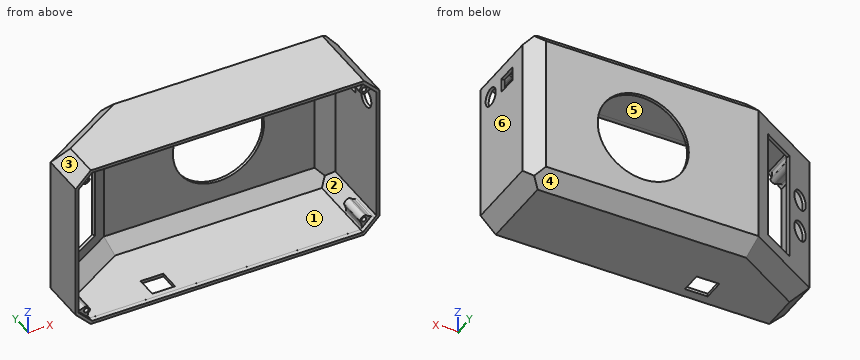
```python
from build123d import *

# Parameters (mm, degrees)
BOSS_EXTRUDE1_DEPTH = 110
CHAMFER1_SIZE       = 10
CHAMFER2_SIZE       = 10
SHELL2_T            = -2
SKETCH2_W           = 25
SKETCH2_H           = 72
CUT_EXTRUDE2_DEPTH  = 90
SKETCH4_R           = 6.5
CUT_EXTRUDE3_DEPTH  = 90
SKETCH5_R           = 1.5
BOSS_EXTRUDE2_DEPTH = 22
FILLET2_R           = 1
CUT_EXTRUDE4_DEPTH  = 3
SKETCH7_R           = 30
CUT_EXTRUDE5_DEPTH  = 61
SKETCH9_R           = 6
SKETCH9_W           = 9.2
SKETCH9_H           = 13
CUT_EXTRUDE6_DEPTH  = 48
SKETCH10_W          = 15
SKETCH10_H          = 14
CUT_EXTRUDE7_DEPTH  = 48


with BuildPart() as part:
    # Sketch1 → Boss-Extrude1 (new body)
    with BuildSketch(Plane.XY):
        Polygon((-200, 30), (-150, 60), (0, 60), (0, 0), (-200, 0), align=None)
    extrude(amount=BOSS_EXTRUDE1_DEPTH)

    # Chamfer1
    chamfer1_edges = [part.edges().sort_by_distance(p)[0] for p in [
        (-175, 45, 110),
        (-200, 15, 110),
        (0, 30, 110),
        (-200, 15, 0),
        (-175, 45, 0),
        (-75, 60, 0),
        (0, 30, 0),
        (-75, 60, 110),
    ]]
    chamfer(chamfer1_edges, length=CHAMFER1_SIZE)

    # Chamfer2
    chamfer2_edges = [part.edges().sort_by_distance(p)[0] for p in [
        (0, 60, 55),
    ]]
    chamfer(chamfer2_edges, length=CHAMFER2_SIZE)

    # Shell2
    shell2_openings = [part.faces().sort_by_distance(p)[0] for p in [
        (-100, 0, 55),
    ]]
    offset(amount=SHELL2_T, openings=shell2_openings, kind=Kind.INTERSECTION)

    # Sketch2 → Cut-Extrude2 (cut)
    with BuildSketch(Plane(origin=(-66.176470588, 110.294117647, 0), x_dir=(0.8574929257125443, 0.5144957554275263, 0), z_dir=(-0.5144957554275263, 0.8574929257125443, 0))):
        with Locations((-120.89691226, -53.994862886)):
            Rectangle(SKETCH2_W, SKETCH2_H)
    extrude(amount=-CUT_EXTRUDE2_DEPTH, mode=Mode.SUBTRACT)

    # Sketch4 → Cut-Extrude3 (cut)
    with BuildSketch(Plane(origin=(-66.176470588, 110.294117647, 0), x_dir=(0.8574929257125443, 0.5144957554275263, 0), z_dir=(-0.5144957554275263, 0.8574929257125443, 0))):
        with Locations(Location((-145.210771321, -43.863127818, 0), (0, 0, 180))):
            Circle(SKETCH4_R)
        with Locations(Location((-145.284101168, -65.939492282, 0), (0, 0, 180))):
            Circle(SKETCH4_R)
    extrude(amount=-CUT_EXTRUDE3_DEPTH, mode=Mode.SUBTRACT)

    # Sketch5 → Boss-Extrude2 (add)
    # profile 1 of 4: a face of its own
    with BuildSketch(Plane.XZ):
        with BuildLine():
            Line((-9.247397896, 106.757043705), (-3.256064459, 100.483765165))
            ThreePointArc((-3.256064459, 100.483765165), (-5.744873038, 99.736713828), (-7.870281401, 98.241757931))
            ThreePointArc((-7.870281401, 98.241757931), (-10.292221795, 99.429108259), (-11.636574356, 101.767550533))
            ThreePointArc((-11.636574356, 101.767550533), (-10.323587398, 104.205602893), (-9.247397896, 106.757043705))
        make_face()
        with Locations((-8.511299496, 101.440505433)):
            Circle(SKETCH5_R, mode=Mode.SUBTRACT)
    # profile 2 of 4: a face of its own
    with BuildSketch(Plane.XZ):
        with BuildLine():
            Line((-10.039510209, 2.683192712), (-3.513368166, 9.046181203))
            ThreePointArc((-3.513368166, 9.046181203), (-5.632030744, 9.88127065), (-7.41571196, 11.29710497))
            ThreePointArc((-7.41571196, 11.29710497), (-9.918845287, 10.389628717), (-11.372165694, 8.158698553))
            ThreePointArc((-11.372165694, 8.158698553), (-10.188591886, 5.546835518), (-10.039510209, 2.683192712))
        make_face()
        with Locations((-8.560298278, 8.510476998)):
            Circle(SKETCH5_R, mode=Mode.SUBTRACT)
    # profile 3 of 4: a face of its own
    with BuildSketch(Plane.XZ):
        with BuildLine():
            Line((-190.1639185, 107.037062189), (-196.90252996, 100.401487601))
            ThreePointArc((-196.90252996, 100.401487601), (-194.442462904, 99.997388644), (-192.214833899, 98.878060765))
            ThreePointArc((-192.214833899, 98.878060765), (-190.200311855, 99.737450982), (-188.807968894, 101.428081542))
            ThreePointArc((-188.807968894, 101.428081542), (-190.20827937, 104.057949981), (-190.1639185, 107.037062189))
        make_face()
        with Locations((-191.50742986, 101.422355381)):
            Circle(SKETCH5_R, mode=Mode.SUBTRACT)
    # profile 4 of 4: a face of its own
    with BuildSketch(Plane.XZ):
        with BuildLine():
            Line((-190.456179178, 3.22389745), (-196.869032371, 9.61475183))
            ThreePointArc((-196.869032371, 9.61475183), (-194.424366222, 10.415493615), (-192.013666474, 11.313328071))
            ThreePointArc((-192.013666474, 11.313328071), (-189.789786951, 9.928723292), (-188.777999187, 7.512309411))
            ThreePointArc((-188.777999187, 7.512309411), (-190.165240448, 5.582610921), (-190.456179178, 3.22389745))
        make_face()
        with Locations((-191.356454927, 8.42171973)):
            Circle(SKETCH5_R, mode=Mode.SUBTRACT)
    extrude(amount=-BOSS_EXTRUDE2_DEPTH)

    # Fillet2
    fillet2_edges = [part.edges().sort_by_distance(p)[0] for p in [
        (-196.80570876, 11, 9.634135884),
        (-190.464527553, 11, 3.292954677),
        (-188.777999187, 11, 7.512309411),
        (-192.013666474, 11, 11.313328071),
        (-10.024061604, 11, 2.80436552),
        (-3.72900082, 11, 9.099426304),
        (-7.41571196, 11, 11.29710497),
        (-11.372165694, 11, 8.158698553),
        (-196.772588823, 11, 100.398984052),
        (-190.174781799, 11, 106.996791076),
        (-192.214833899, 11, 98.878060765),
        (-188.807968894, 11, 101.428081542),
        (-3.305525067, 11, 100.477097942),
        (-9.339081083, 11, 106.510653959),
        (-11.636574356, 11, 101.767550533),
        (-7.870281401, 11, 98.241757931),
    ]]
    fillet(fillet2_edges, radius=FILLET2_R)

    # Sketch6 → Cut-Extrude4 (cut)
    with BuildSketch(Plane.XZ):
        Polygon((-198.003014977, 10.842085531), (-189.211900871, 1.9947291), (-10.828081787, 1.9947291), (-2.004701189, 10.828504844), (-2.004701189, 99.205715336), (-10.87289136, 108.000350983), (-189.173255871, 108.000350983), (-198.003014977, 99.184415132), align=None)
    extrude(amount=-CUT_EXTRUDE4_DEPTH, mode=Mode.SUBTRACT)

    # Sketch7 → Cut-Extrude5 (cut)
    with BuildSketch(Plane(origin=(0, 60, 0), x_dir=(1, 0, 0), z_dir=(0, 1, 0))):
        with Locations(Location((-74.048474832, -53.651868822, 0), (0, 0, 180))):
            Circle(SKETCH7_R)
    extrude(amount=-CUT_EXTRUDE5_DEPTH, mode=Mode.SUBTRACT)

    # Sketch9 → Cut-Extrude6 (cut)
    with BuildSketch(Plane(origin=(0, 0, 0), x_dir=(0, 0, -1), z_dir=(1, 0, 0))):
        with Locations((-87.253164056, 12.081575525)):
            Circle(SKETCH9_R)
        with Locations((-87.170080289, 31.378854617)):
            Rectangle(SKETCH9_W, SKETCH9_H)
    extrude(amount=-CUT_EXTRUDE6_DEPTH, mode=Mode.SUBTRACT)

    # Sketch10 → Cut-Extrude7 (cut)
    with BuildSketch(Plane(origin=(0, 0, 0), x_dir=(-1, 0, 0), z_dir=(0, 0, -1))):
        with Locations((138.565692725, 13.322096046)):
            Rectangle(SKETCH10_W, SKETCH10_H)
    extrude(amount=-CUT_EXTRUDE7_DEPTH, mode=Mode.SUBTRACT)


solid = part.part
```
The model under review builds one solid part; all positions refer to its coordinate system, in mm. Face numbers are marked on the shaded views. A direction names the side the tool comes from. Round coordinates to 2 decimals unless told otherwise and drop trailing zeros.
Item 1: Take a section at B-B (z = 63). Give the number of separate pieces and of enclosed holes in the cut face, then the cut area to 3 significant figures.
Determined:
separate pieces: 4
enclosed holes: 0
area: 391 mm2
Item 2: Clearance check with flat-ended pins moving along their axes: pin 1 Ø7 at (x, z) = (-9.5, 101.5) entering from +Y; pin 2 Ø2.5 at (x, z) = (-8.56, 8.51) entering from +Y; pin 3 Ø2.5 at (x, z) = (-193, 105) entering from +Y; pin 4 Ø1.6 at (x, z) = (-142, 1) entering from +Y. State where each tip first meets the part, or that it passes through.
Determined:
pin 1: stops at y = 60
pin 2: stops at y = 59.42
pin 3: stops at y = 30.01
pin 4: stops at y = 51.8
Item 3: For the marked faces 1, 2 and 3, list the 3-axis set-ups (+Z, -Z, +X, -X, +Y, -Y) from which the entire face can be reached by the end or side of a thin tool; tool diameter is ignored.
Determined:
face 1: -Y
face 2: none
face 3: +Z, -X, +Y, -Y
Item 4: For line 1 (Z direction, x = -131.5, y = 39.5); line 2 (X direction, y = 25.5, z = 98); line 3 (Z direction, x = -140, y = 52), list the stretches that pass through material, from the lowest coordinate up.
Determined:
line 1: z = 0 to 2, 108 to 110
line 2: x = -200 to -198, -2 to 0
line 3: z = 2 to 4.83, 105.17 to 108
Item 5: Mouldability with a two-part tool opening along X and no side actions: class the marked faces 4, 5 and 6 as released by +X, released by -X, zero draft, split by the parting line, or undercut.
Determined:
face 4: zero draft
face 5: undercut
face 6: released by +X
